Build history of the part. All positions in model axes, mm. A direction names the side the tool comes from. Coordinates: 2 decimals unless noted, no trailing zeros. Order: outer loops, then holes, each group sorted by start corner. A loop starts at its lowest first (then second) coordinate and runs counter-clockwise, first axis right, second up. Notation, with made-up numbers: (19.25, -10.5) - (33.25, -10.5) arc R30 cw to (33.25, 16.5) - close; hole circle Ø5 at (67.5, -29). An arc over 180 degrees is marked (long way). Return JSON: item names as keys, results as strings.
from build123d import *

# Parameters (mm, degrees)
F0_R     = 39.39632
F1_DEPTH = 25.4


with BuildPart() as f1:
    # F0 (on Top) → F1 (new body)
    with BuildSketch(Plane.XY):
        Circle(F0_R)
        Polygon((-12.259586, -12.635498), (-12.259586, 0), (-12.259586, 12.635498), (0, 12.635498), (12.259586, 12.635498), (12.259586, 0), (12.259586, -12.635498), (0, -12.635498), align=None, mode=Mode.SUBTRACT)
    extrude(amount=F1_DEPTH)


solid = f1.part
1. Probe L1, parallel to X at y = 3, z = 23.5; L2, parallel to Y at x = -8, z = 23.5; L3, parallel to Y at x = 9, z = 2.75. List the from-to ranges inside material, lowest first.
Check values:
{"L1": "-39.28 to -12.26, 12.26 to 39.28", "L2": "-38.58 to -12.64, 12.64 to 38.58", "L3": "-38.35 to -12.64, 12.64 to 38.35"}
2. Cut at A-A on x = 0. Give the cut face in (y, z).
Check values:
{"outline": "(-39.4, 0) - (-12.64, 0) - (-12.64, 25.4) - (-39.4, 25.4) - close; (12.64, 0) - (39.4, 0) - (39.4, 25.4) - (12.64, 25.4) - close"}
3. Cut at D-D on y = -30. Give the cut face in (x, z).
Check values:
{"outline": "(-25.54, 0) - (25.54, 0) - (25.54, 25.4) - (-25.54, 25.4) - close"}
4. Cut at C-C on z = 19.5. Give the cut face in (x, y).
Check values:
{"outline": "circle Ø78.79 at (0, 0); hole (-12.26, -12.64) - (12.26, -12.64) - (12.26, 12.64) - (-12.26, 12.64) - close"}
5. Mould opens along X. For faces 3 (the flat face through (17, 1, 0)), 4 (the cylindrical face through (37.58, 11.83, 12.52)), 5 (the flat face through (-12.26, 0, 13)) say: pulls with the +X half, pulls with the -X half, needs draft (parallel to the pull), parting line crosses it, or undercut.
Check values:
{"face 3": "needs draft", "face 4": "parting line crosses it", "face 5": "undercut"}
6. Drop flat-ended pins along their axis: pin 1 (4 mm diameter, centred on x = 18.5, z = 6, fed in from -Y); pin 2 (12.5 mm diameter, centred on x = -4.5, z = 12.5, fed in from +Y); pin 3 (4 mm diameter, centred on y = -21.5, z = 3.5, fed in from +X). Give the stop position or say it passes through.
Check values:
{"pin 1": "y = -35.77", "pin 2": "y = 39.4", "pin 3": "x = 34.23"}
7. Cut at B-B on y = 0. Give the cut face in (x, z), plus the area to 3 significant figures.
Check values:
{"outline": "(-39.4, 0) - (-12.26, 0) - (-12.26, 25.4) - (-39.4, 25.4) - close; (12.26, 0) - (39.4, 0) - (39.4, 25.4) - (12.26, 25.4) - close", "area": "1,380 mm²"}
8. Tool access for faces 1 (the flat face through (17, 1, 25.4)), 2 (the flat face through (12.26, 0, 13)): list every direction of +Z, -Z, +X, -X, +Y, -Y with a clear straight run to the whole face (end or side of a thin tool).
Check values:
{"face 1": "+Z, +X, -X, +Y, -Y", "face 2": "+Z, -Z"}
